Answer from the drawing. Dimensions are ordinates in mm from the lowest x, y and z of the part. A direction names the side the tool comes from. Give positions to 0.01 mm unless a question says otherwise; leave off trailing zeros. Order: outer loops, then holes, each group sorted by start corner. A loop starts at its lowest first (then second) coordinate and runs counter-clockwise, first axis right, second up. Notation, with made-up numbers: (21, -30) - (78, -30) arc R20 ccw to (78, -23) - close; hole circle Ø9 at (19.5, -6). An arc over 180 degrees is marked (long way). Answer in a Markdown table with one row per item. Add a question column.
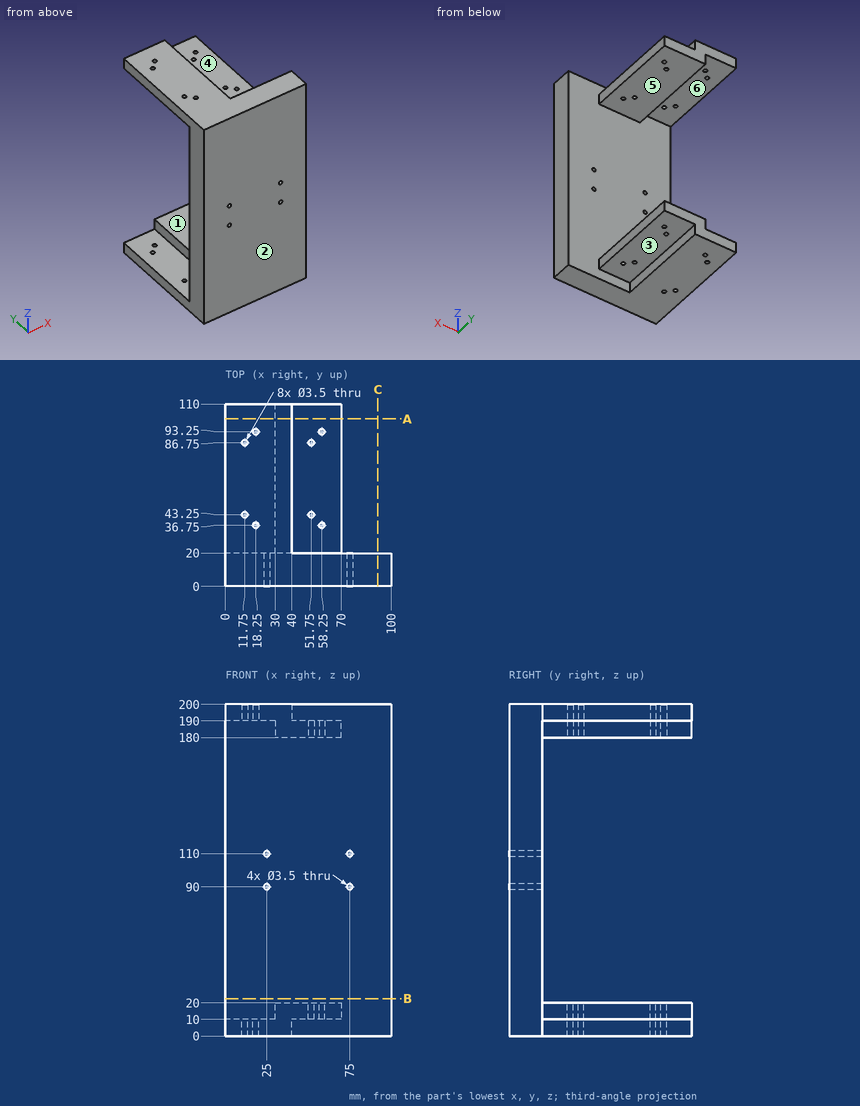
(1) Find section C-C, the plane x = 92. Write down the section's boundary in (y, z).
(2) Straight lines are drawn through the part: line 1 (Y direction, x = 58.25, z = 183.25); line 2 (Y direction, x = 51.75, z = 187.5); line 3 (Z direction, x = 75, y = 15.25). For each, find the intervals that lie inside material, in ascending order.
(3) Find section A-A, the plane y = 101. Write down the section's boundary in (x, z), plus the area to 3 significant figures.
(4) For the marked faces 4, 5 and 6, determine the directions among +Z, -Z, +X, -X, +Y, -Y from which every point of the face is accessible in a straight line to the end or side of a thin tool.
(5) The mould has two halves that part along Z. Classify the marked faces 1, 2 and 3: +Z half, -Z half, draft (parallel to the pull), parting line (faces both ways), or undercut.
(6) Each of these flat-tipped pins is pushed along its axis until it touches: P1, Ø8, axis at y = 68.5, z = 187, coming from the +X side; P2, Ø24, axis at x = 16, y = 71.5, coming from the -Z side; P3, Ø4, axis at x = 58.25, y = 93.25, coming from the +Z side; P4, Ø6, axis at x = 28.5, z = 130.5, coming from the +Y side. Where does it stop, or does it pass through?
(7) Find section B-B, the plane z = 22.5. Write down the section's boundary in (x, y), plus the area to 3 significant figures.
Answer key:
| question | item | result |
|---|---|---|
| 1 | outline | (0, 0) - (20, 0) - (20, 200) - (0, 200) - close |
| 2 | line 1 | 0 to 35, 38.5 to 91.5, 95 to 110 |
| 2 | line 2 | 0 to 41.5, 45 to 85, 88.5 to 110 |
| 2 | line 3 | 0 to 88.25, 91.75 to 108.25, 111.75 to 200 |
| 3 | outline | (0, 0) - (40, 0) - (40, 10) - (70, 10) - (70, 20) - (30, 20) - (30, 10) - (0, 10) - close; (0, 190) - (30, 190) - (30, 180) - (70, 180) - (70, 190) - (40, 190) - (40, 200) - (0, 200) - close |
| 3 | area | 1,600 mm² |
| 4 | face 4 | +Z, +X, +Y |
| 4 | face 5 | +X, -X, +Y |
| 4 | face 6 | -X, +Y |
| 5 | face 1 | undercut |
| 5 | face 2 | draft |
| 5 | face 3 | -Z half |
| 6 | P1 | x = 70 |
| 6 | P2 | z = 0 |
| 6 | P3 | z = 190 |
| 6 | P4 | y = 20 |
| 7 | outline | (0, 0) - (100, 0) - (100, 20) - (0, 20) - close |
| 7 | area | 2,000 mm² |
